Source: CAD feature listing. Evaluate the final solid. Frame: model axes, mm. A direction names the side the tool comes from. Round coordinates to 2 decimals unless told otherwise and drop trailing zeros.
(1) First-contact query: pin 1 Ø1 at (x, z) = (-23, -70.5) entering from -Y. Flat tip, straight axial feed; report the tip coordinate or a pass-through.
(2) Section A-A, the plane y = 1.6. Count the separate pieces of the cut face and the enclosed holes in it, plus the area to 3 significant figures.
(3) Mould query, pull axis X, two halves, no side actions, for faces 6 (the cylindrical face through (-35, 3, -21)), 7 (the flat face through (0, 2, -234)), 8 (the flat face through (-30, 3, -24)), 9 (the flat face through (-57, 5, -119)). Classes: pulls with the +X half, pulls with the -X half, needs draft (parallel to the pull), parting line crosses it, or undercut.
(4) Set-up query: faces 1 (the flat face through (-13.91, 2.54, -222.57)), 2 (the flat face through (-57, 0, -119)), 3 (the flat face through (0, 2, -104)), 4 (the flat face through (-30, 3, -18)), 5 (the flat face through (-106, 3, -91.5)). Return all of +Z, -Z, +X, -X, +Y, -Y with unobstructed straight access to the full face (end or side cutting, diameter ignored); none if empty.
(5) Material intervals for probe 1 along Z at (x, y) = (-84.2, 1.6); probe 2 along Z at (x, y) = (-43, 3.8); probe 3 along X at (y, z) = (2.6, -234), sorted ascending.
Autodesk Inventor part; units mm, degrees
ref_plane "YZ Plane" through (0, 0, 0) normal (1, 0, 0) x (0, 1, 0)
ref_plane "XZ Plane" through (0, 0, 0) normal (0, 1, 0) x (-1, 0, 0)
ref_plane "XY Plane" through (0, 0, 0) normal (0, 0, 1) x (1, 0, 0)
sketch "Sketch1" plane through (0, 0, 0) normal (0, 1, 0) x (-1, 0, 0)
  line L0 (0, 0) -> (116.2, 0)
  line L1 (116.2, 0) -> (116.2, -242)
  line L2 (116.2, -242) -> (0, -242)
  line L3 (0, -242) -> (0, 0)
  dimension "d0" = 116.2
  dimension "d1" = 242
extrude "Extrusion1" add sketch "Sketch1" along normal blind 5
sketch "Sketch2" plane through (0, 5, 0) normal (0, 1, 0) x (1, 0, 0)
  line L0 (-43, 8) -> (-12, 8) construction
  line L1 (-12, 8) -> (-12, 234) construction
  line L2 (-12, 234) -> (-43, 234) construction
  line L3 (-43, 234) -> (-43, 8) construction
  line L4 (-116.2, 0) -> (0, 0) construction
  line L5 (0, 242) -> (-116.2, 242) construction
  line L6 (0, 0) -> (0, 242) construction
  dimension "d4" = 8
  dimension "d5" = 8
  dimension "d6" = 12
  dimension "d7" = 31
hole "Hole1" at (-12, 5, -8) at (-43, 5, -8) at (-43, 5, -234) at (-12, 5, -234) direction (0, -1, 0) diameter 3.8 end through all
sketch "Sketch3" plane through (0, 5, 0) normal (0, 1, 0) x (1, 0, 0)
  line L0 (-128.5064, 215.5) -> (22.7754, 215.5) construction
  line L1 (0, 242) -> (-116.2, 242)
  line L2 (0, 225.5) -> (-18, 225.5)
  line L3 (-18, 225.5) -> (-18, 205.5)
  line L4 (-18, 205.5) -> (0, 205.5)
  line L5 (0, 205.5) -> (0, 225.5)
  line L6 (0, 225.5) -> (-18, 205.5) construction
  line L7 (-18, 225.5) -> (0, 205.5) construction
  line L8 (0, 0) -> (0, 242)
  line L9 (-18, 211.5) -> (-10, 205.5)
  line L10 (-18, 219.5) -> (-10, 225.5)
  point P0 (-9, 215.5)
  point P1 (-18, 215.5)
  dimension "d15" = 26.5
  dimension "d16" = 20
  dimension "d17" = 18
  dimension "d18" = 8
  dimension "d19" = 10
extrude "Extrusion2" cut sketch "Sketch3" against normal through all contours L5 L4 L9 L3 L10 L2
fillet "Fillet1" radius 2 4 edges at (-18, 2.5, -219.5) (-10, 2.5, -225.5) (-18, 2.5, -211.5) (-10, 2.5, -205.5)
sketch "Sketch4" plane through (0, 5, 0) normal (0, 1, 0) x (1, 0, 0)
  line L0 (-84.2, 269.0758) -> (-84.2, -69.3617) construction
  line L1 (0, 0) -> (0, 205.5) construction
  line L2 (-116.2, 0) -> (0, 0) construction
  line L3 (0, 242) -> (-116.2, 242) construction
  line L4 (-116.2, 242) -> (-116.2, 0)
  line L5 (-60, 78.142) -> (-60, -51.5949) construction
  point P0 (-84.2, 223)
  point P1 (-84.2, 211)
  point P2 (-60, 24)
  point P3 (-60, 12)
  dimension "d24" = 12
  dimension "d25" = 12
  dimension "d26" = 12
  dimension "d27" = 31
  dimension "d35" = 32
  dimension "d36" = 60
hole "Hole2" at (-84.2, 5, -223) at (-84.2, 5, -211) at (-60, 5, -24) at (-60, 5, -12) direction (0, -1, 0) diameter 3.8 end through all
sketch "Sketch5" plane through (0, 5, 0) normal (0, 1, 0) x (1, 0, 0)
  line L0 (-116.2, 242) -> (-116.2, 0)
  line L1 (-116.2, 0) -> (0, 0)
  point P0 (-100.2, 23.25)
  dimension "d37" = 16
  dimension "d38" = 23.25
hole "Hole3" at (-100.2, 5, -23.25) direction (0, -1, 0) diameter 3.8 end through all
sketch "Sketch6" plane through (0, 5, 0) normal (0, 1, 0) x (1, 0, 0)
  line L0 (-109.7, 280.0258) -> (-109.7, -41.1522) construction
  line L1 (-116.2, 242) -> (-116.2, 0)
  line L2 (0, 242) -> (-116.2, 242)
  point P0 (0, 0)
  point P1 (-109.7, 234)
  point P2 (-109.7, 22.25)
  dimension "d46" = 6.5
  dimension "d47" = 8
  dimension "d48" = 211.75
hole "Hole4" at (-109.7, 5, -234) at (-109.7, 5, -22.25) direction (0, -1, 0) diameter 3.8 end through all
sketch "Sketch7" plane through (0, 5, 0) normal (0, 1, 0) x (1, 0, 0)
  line L0 (-50.7253, 21) -> (31.7934, 21) construction
  line L1 (-116.2, 0) -> (0, 0) construction
  line L2 (-32, 24) -> (-27.5, 24)
  line L3 (-25, 21.5) -> (-25, 20.5)
  line L4 (-27.5, 18) -> (-32, 18)
  line L5 (-32, 18) -> (-32, 21)
  line L6 (-32, 24) -> (-25, 18) construction
  line L7 (-25, 24) -> (-32, 18) construction
  line L8 (0, 0) -> (0, 205.5) construction
  arc A0 (-32, 24) -> (-32, 18) centre (-32, 21) ccw
  arc A1 (-25, 21.5) -> (-27.5, 24) centre (-27.5, 21.5) ccw
  arc A2 (-27.5, 18) -> (-25, 20.5) centre (-27.5, 20.5) ccw
  point P0 (-28.5, 21)
  dimension "d56" = 21
  dimension "d57" = 7
  dimension "d58" = 6
  dimension "d59" = 25
  dimension "d62" = 2.5
extrude "Extrusion3" cut sketch "Sketch7" against normal blind 10
sketch "Sketch8" plane through (0, 5, 0) normal (0, 1, 0) x (1, 0, 0)
  line L0 (-195.7233, 114) -> (78.1714, 114) construction
  line L1 (-116.2, 0) -> (0, 0)
  line L2 (-136.2, 91.5) -> (-96.2, 91.5)
  line L3 (-96.2, 91.5) -> (-96.2, 136.5)
  line L4 (-96.2, 136.5) -> (-136.2, 136.5)
  line L5 (-136.2, 136.5) -> (-136.2, 91.5)
  line L6 (-116.2, 242) -> (-116.2, 0)
  line L7 (-136.2, 91.5) -> (-96.2, 136.5) construction
  line L8 (-96.2, 91.5) -> (-136.2, 136.5) construction
  point P0 (-116.2, 114)
  point P1 (-116.2, 136.5)
  point P2 (-116.2, 91.5)
  dimension "d63" = 114
  dimension "d64" = 40
  dimension "d65" = 45
extrude "Extrusion4" cut sketch "Sketch8" against normal through all contours L6 L4 L3 L2
fillet "Fillet2" radius 4 4 edges at (-116.2, 2.5, -136.5) (-116.2, 2.5, -91.5) (-96.2, 2.5, -91.5) (-96.2, 2.5, -136.5)
fillet "Fillet3" radius 2 1 edges at (-116.2, 2.5, -242)
properties part number "Battery Side Plate"
Output values:
1. pin 1: stops at y = 0
2. separate pieces: 1
2. enclosed holes: 12
2. area: 26,700 mm2
3. face 6: undercut
3. face 7: pulls with the +X half
3. face 8: undercut
3. face 9: needs draft
4. face 1: +X, +Y, -Y
4. face 2: +Z, -Z, +X, -X, -Y
4. face 3: +Z, -Z, +X, +Y, -Y
4. face 4: +Y, -Y
4. face 5: -X, +Y, -Y
5. probe 1: z = -242 to -224.9, -221.1 to -212.9, -209.1 to 0
5. probe 2: z = -242 to -235.9, -232.1 to -9.9, -6.1 to 0
5. probe 3: x = -116.2 to -111.6, -107.8 to -44.9, -41.1 to -13.9, -10.1 to 0
